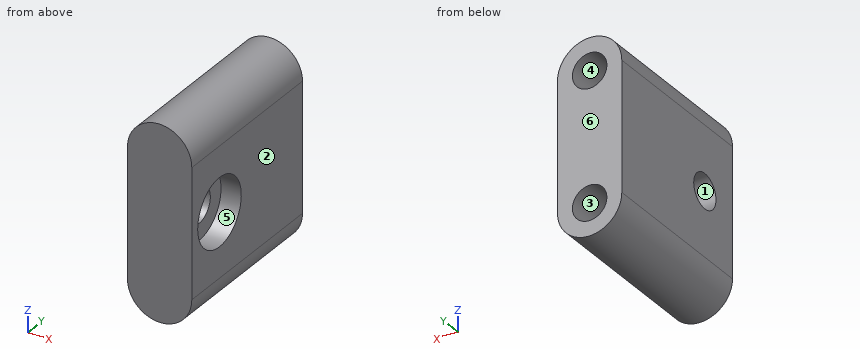
```python
from build123d import *

# Parameters (mm, degrees)
SKETCH8_W                   = 15.875
SKETCH8_H                   = 38.1
BOSS_EXTRUDE2_DEPTH         = 25.4
F_1_4_20_TAPPED_HOLE1_D     = 5.1054
F_1_4_20_TAPPED_HOLE1_DEPTH = 16.51
F_1_4_20_TAPPED_HOLE1_TIP   = 1.533816902
SKETCH10_W                  = 15.875
SKETCH10_H                  = 38.1
CUT_EXTRUDE2_DEPTH          = 26.4
CUT_EXTRUDE5_START          = -19.05
SKETCH13_R                  = 5.000000033
SKETCH13_R_2                = 3.175
CUT_EXTRUDE5_DEPTH          = 3
F_1_4_20_TAPPED_HOLE2_D     = 5.1054
F_1_4_20_TAPPED_HOLE2_DEPTH = 16.51
F_1_4_20_TAPPED_HOLE2_TIP   = 1.533816902


with BuildPart() as part:
    # Sketch8 → Boss-Extrude2 (new body)
    with BuildSketch(Plane(origin=(0, 0, 0), x_dir=(1, 0, 0), z_dir=(0, 1, 0))):
        with Locations((-23.8125, 0)):
            Rectangle(SKETCH8_W, SKETCH8_H)
    extrude(amount=BOSS_EXTRUDE2_DEPTH)

    # 1/4-20 Tapped Hole1
    with Locations(Plane(origin=(0, 25.4, 0), x_dir=(1, 0, 0), z_dir=(0, 1, 0))):
        with Locations((-23.8125, 9.525), (-23.8125, -9.525)):
            Hole(F_1_4_20_TAPPED_HOLE1_D / 2, depth=F_1_4_20_TAPPED_HOLE1_DEPTH)
            with Locations((0, 0, -(F_1_4_20_TAPPED_HOLE1_DEPTH + F_1_4_20_TAPPED_HOLE1_TIP / 2))):  # 118° drill point
                Cone(0, F_1_4_20_TAPPED_HOLE1_D / 2, F_1_4_20_TAPPED_HOLE1_TIP, mode=Mode.SUBTRACT)

    # Sketch10 → Cut-Extrude2 (cut, through all)
    with BuildSketch(Plane(origin=(0, 0, 0), x_dir=(1, 0, 0), z_dir=(0, 1, 0))):
        with Locations((-23.8125, 0)):
            Rectangle(SKETCH10_W, SKETCH10_H)
        with BuildLine():
            Line((-28.575, 9.525), (-28.575, -9.525))
            ThreePointArc((-28.575, -9.525), (-23.8125, -14.2875), (-19.05, -9.525))
            Line((-19.05, -9.525), (-19.05, 9.525))
            ThreePointArc((-19.05, 9.525), (-23.8125, 14.2875), (-28.575, 9.525))
        make_face(mode=Mode.SUBTRACT)
    extrude(amount=CUT_EXTRUDE2_DEPTH, mode=Mode.SUBTRACT)

    # Sketch13 → Cut-Extrude5 (cut)
    with BuildSketch(Plane(origin=(0, 0, 0), x_dir=(0, 0, -1), z_dir=(1, 0, 0)).offset(CUT_EXTRUDE5_START)):
        with Locations((0, 6.35)):
            Circle(SKETCH13_R)
        with Locations((0, 6.35)):
            Circle(SKETCH13_R_2, mode=Mode.SUBTRACT)
        with Locations((0, 6.35)):
            Circle(SKETCH13_R_2)
    extrude(amount=-CUT_EXTRUDE5_DEPTH, mode=Mode.SUBTRACT)

    # 1/4-20 Tapped Hole2
    with Locations(Plane(origin=(-19.05, 0, 0), x_dir=(0, 0, -1), z_dir=(1, 0, 0))):
        with Locations((0, 6.35)):
            Hole(F_1_4_20_TAPPED_HOLE2_D / 2, depth=F_1_4_20_TAPPED_HOLE2_DEPTH)
            with Locations((0, 0, -(F_1_4_20_TAPPED_HOLE2_DEPTH + F_1_4_20_TAPPED_HOLE2_TIP / 2))):  # 118° drill point
                Cone(0, F_1_4_20_TAPPED_HOLE2_D / 2, F_1_4_20_TAPPED_HOLE2_TIP, mode=Mode.SUBTRACT)


solid = part.part
```
Could you check a few things on this model? Use its own coordinates, in mm. Face numbers are marked on the shaded views. A direction names the side the tool comes from. Coordinates: 2 decimals unless noted, no trailing zeros. Write each loop counter-clockwise with the first axis right and the second up, starting at its lowest first coordinate (ties: lowest second). Pieces come first, ordered by that corner, then holes. Notation, with made-up numbers: M 51.5,-7.75 L 82.5,-7.75 A32 ccw 82.5,22.25 Z; hole C -21,37.5 d10. An arc over 180 degrees is marked long. Answer as CSV lines item,"result". Start each with the question number.
1) I want a section at C-C, the plane y = 10.5. Give the number of separate pieces and of enclosed holes in the cut face, and give its area (3 significant figures).
2) For P1, Ø8, axis at y = 6.35, z = 0, coming from the +X side; P2, Ø1.5, axis at x = -26.5, y = 7.5, coming from the -Z side; P3, Ø4, axis at x = -23.81, z = 9.52, coming from the +Y side, each with a flat end and sliding along its axis, tell me the tip position at first contact or that it passes through.
3) I want a section at B-B, the plane z = 0. Please give me the cut outline in (x, y) (3 decimals), and give its area (3 significant figures).
4) Please list where these lines run through material, in increasing order: line 1 (Z direction, x = -22.25, y = 11.75); line 2 (Y direction, x = -27.5, z = -1); line 3 (Z direction, x = -25, y = 16.5). Write a range as from..to.
5) We'd pull the mould along X, two halves only. Please class the marked faces 1, 2 and 3: +X half, -X half, draft (parallel to the pull), parting line (faces both ways), or undercut.
6) I want a section at D-D, the plane x = -27.5. Please give me the cut outline in (y, z).
7) For the marked faces 4, 5 and 6, which set-ups out of +Z, -Z, +X, -X, +Y, -Y let a thin tool reach every point of the face, with its end or its side?
Data:
1,separate pieces,"1"
1,enclosed holes,"2"
1,area,"195 mm^2"
2,P1,"stops at x = -22.05"
2,P2,"stops at z = -13.88"
2,P3,"stops at y = 8.56"
3,outline,"M -28.575,0 L -19.05,0 L -19.05,1.35 L -22.05,1.35 L -22.05,3.797 L -28.575,3.797 Z; M -28.575,8.903 L -22.05,8.903 L -22.05,11.35 L -19.05,11.35 L -19.05,25.4 L -28.575,25.4 Z"
3,area,"179 mm^2"
4,line 1,"z = -14.02..-11.54, -7.51..7.51, 11.54..14.02"
4,line 2,"y = 0..4, 8.7..25.4"
4,line 3,"z = -14.14..-11.78, -7.27..7.27, 11.78..14.14"
5,face 1,"draft"
5,face 2,"+X half"
5,face 3,"undercut"
6,outline,"M 0,-12.54 L 25.4,-12.54 L 25.4,12.54 L 0,12.54 Z; hole C 6.35,0 d5.11"
7,face 4,"+Y"
7,face 5,"+X"
7,face 6,"+Z, -Z, +X, -X, +Y"
